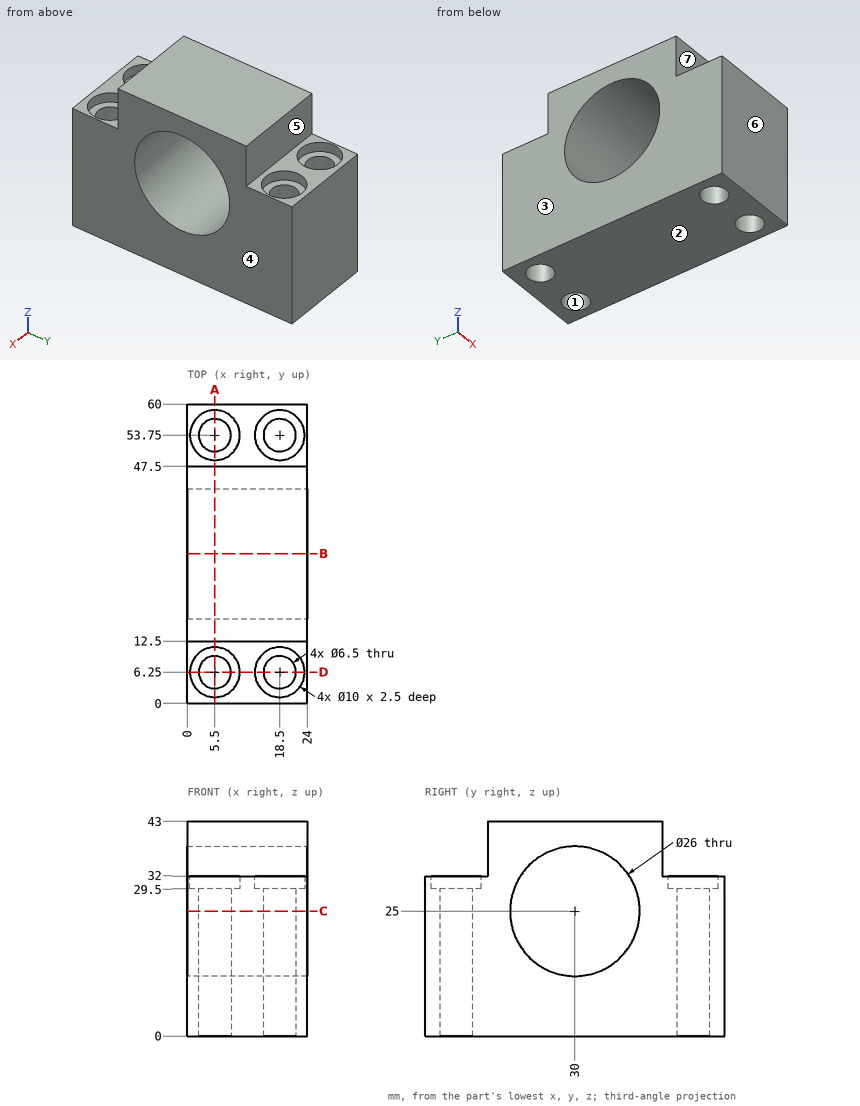
Can you work these out from the drawing? Everything is in mm from the part's minimum corner. A direction names the side the tool comes from. Give positions to 0.01 mm unless a question says otherwise; leave off trailing zeros. Write each loop counter-clockwise with the first axis right and the second up, starting at its lowest first coordinate (ties: lowest second). Pieces come first, ordered by that corner, then holes. Notation, with made-up numbers: (71, 67) -> (87, 67) arc R25 cw to (87, 84) -> close; hole circle Ø11 at (58, 64.5). An arc over 180 degrees is marked (long way). Write each question's results on one line, items separated by ' | '. Start each with the question number.
Q1. Which directions (+Z, -Z, +X, -X, +Y, -Y) give clear straight access to the entire face, cutting with the end or side of a thin tool? Please do the marked faces 5, 6 and 7.
Q2. We'd pull the mould along X, two halves only. Please class the marked faces 1, 2, 3 and 4: +X half, -X half, draft (parallel to the pull), parting line (faces both ways), or undercut.
Q3. Suppose I cut it at C-C, the plane z = 25. List the corners of the cut face in (x, y) for me.
Q4. Suppose I cut it at B-B, the plane y = 30. List the corners of the cut face in (x, z) for me.
Q5. Suppose I cut it at A-A, the plane x = 5.5. List the corners of the cut face in (y, z) for me.
Q6. I'm going to push flat-ended pins straight in: pin 1 Ø11 at (x, y) = (19.5, 5) entering from +Z; pin 2 Ø7.5 at (x, y) = (5.5, 6.25) entering from -Z; pin 3 Ø5 at (x, y) = (5, 53.5) entering from -Z; pin 4 Ø8.5 at (x, y) = (18.5, 6.25) entering from +Z. Where does each tip first touch, or does it pass through?
Q7. I need wall thicknesses on probe 1 along Y at (x, z) = (5.5, 8.25); probe 2 along X at (y, z) = (6, 18); probe 3 along X at (y, z) = (6, 30). Which ranges of each line are inside material? Lowest first, please.
Q8. Suppose I cut it at D-D, the plane y = 6.25. List the corners of the cut face in (x, z) for me, and give its area (4 significant figures).
Outcome:
1) face 5: +Z, +X, -X, +Y | face 6: +Z, -Z, +X, -X, -Y | face 7: +Z, +X, -X, -Y
2) face 1: undercut | face 2: draft | face 3: -X half | face 4: +X half
3) outline: (0, 0) -> (24, 0) -> (24, 17) -> (0, 17) -> close; (0, 43) -> (24, 43) -> (24, 60) -> (0, 60) -> close; hole circle Ø6.5 at (5.5, 6.25); hole circle Ø6.5 at (5.5, 53.75); hole circle Ø6.5 at (18.5, 6.25); hole circle Ø6.5 at (18.5, 53.75)
4) outline: (0, 0) -> (24, 0) -> (24, 12) -> (0, 12) -> close; (0, 38) -> (24, 38) -> (24, 43) -> (0, 43) -> close
5) outline: (0, 0) -> (3, 0) -> (3, 29.5) -> (1.25, 29.5) -> (1.25, 32) -> (0, 32) -> close; (9.5, 0) -> (50.5, 0) -> (50.5, 29.5) -> (48.75, 29.5) -> (48.75, 32) -> (47.5, 32) -> (47.5, 43) -> (12.5, 43) -> (12.5, 32) -> (11.25, 32) -> (11.25, 29.5) -> (9.5, 29.5) -> close; (57, 0) -> (60, 0) -> (60, 32) -> (58.75, 32) -> (58.75, 29.5) -> (57, 29.5) -> close; hole circle Ø26 at (30, 25)
6) pin 1: z = 32 | pin 2: z = 0 | pin 3: through | pin 4: z = 29.5
7) probe 1: 0 to 3, 9.5 to 50.5, 57 to 60 | probe 2: 0 to 2.26, 8.74 to 15.26, 21.74 to 24 | probe 3: 0 to 0.51, 10.49 to 13.51, 23.49 to 24
8) outline: (0, 0) -> (2.25, 0) -> (2.25, 29.5) -> (0.5, 29.5) -> (0.5, 32) -> (0, 32) -> close; (8.75, 0) -> (15.25, 0) -> (15.25, 29.5) -> (13.5, 29.5) -> (13.5, 32) -> (10.5, 32) -> (10.5, 29.5) -> (8.75, 29.5) -> close; (21.75, 0) -> (24, 0) -> (24, 32) -> (23.5, 32) -> (23.5, 29.5) -> (21.75, 29.5) -> close | area: 334.5 mm2
